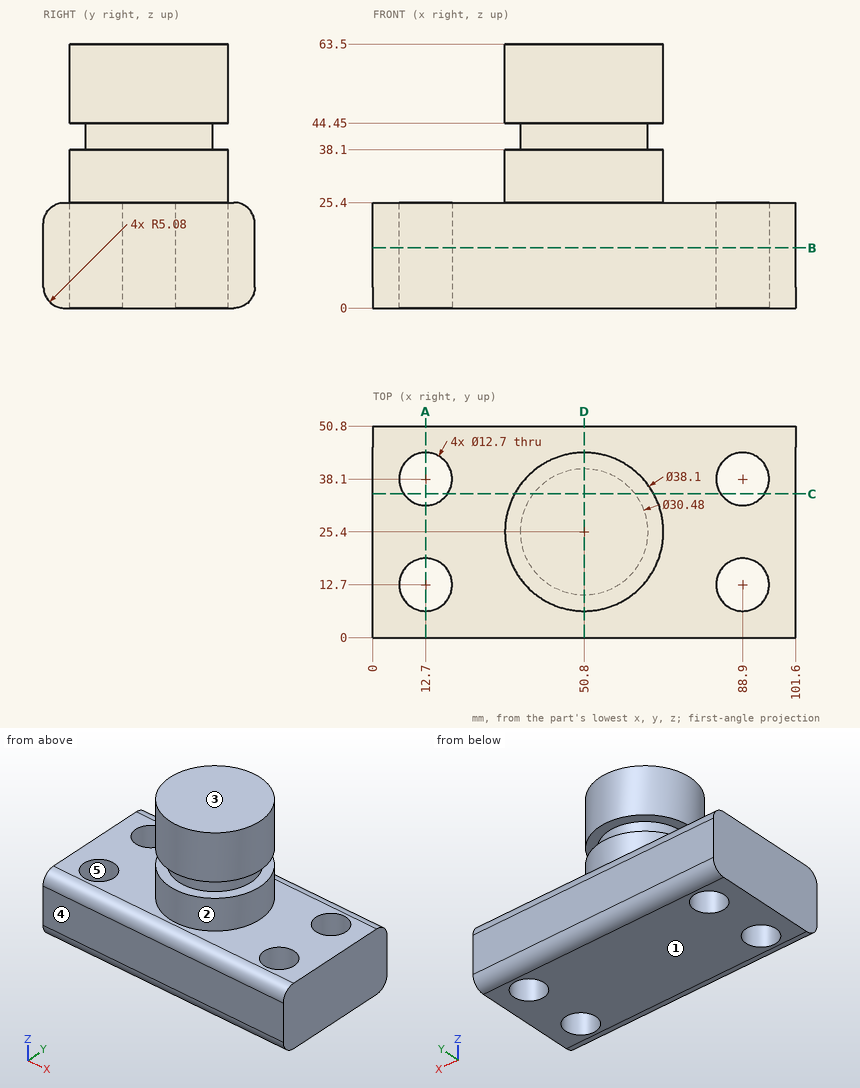
Drawing for the job (mm, zero at the part's lowest x, y, z). A direction names the side the tool comes from. Coordinates: 2 decimals unless noted, no trailing zeros. Order: outer loops, then holes, each group sorted by start corner. A loop starts at its lowest first (then second) coordinate and runs counter-clockwise, first axis right, second up.
Item 1: Band-saw the part on B-B on z = 14.5. List the corners of the cut face in (x, y).
Check sheet entries:
outline: (0, 0) - (101.6, 0) - (101.6, 50.8) - (0, 50.8) - close; hole circle Ø12.7 at (12.7, 12.7); hole circle Ø12.7 at (12.7, 38.1); hole circle Ø12.7 at (88.9, 12.7); hole circle Ø12.7 at (88.9, 38.1)
Item 2: Band-saw the part on A-A on x = 12.7. List the corners of the cut face in (y, z), plus the area to 3 significant figures.
Check sheet entries:
outline: (0, 5.08) arc R5.08 ccw to (5.08, 0) - (6.35, 0) - (6.35, 25.4) - (5.08, 25.4) arc R5.08 ccw to (0, 20.32) - close; (19.05, 0) - (31.75, 0) - (31.75, 25.4) - (19.05, 25.4) - close; (44.45, 0) - (45.72, 0) arc R5.08 ccw to (50.8, 5.08) - (50.8, 20.32) arc R5.08 ccw to (45.72, 25.4) - (44.45, 25.4) - close
area: 623 mm2
Item 3: Band-saw the part on D-D on x = 50.8. List the corners of the cut face in (y, z).
Check sheet entries:
outline: (0, 5.08) arc R5.08 ccw to (5.08, 0) - (45.72, 0) arc R5.08 ccw to (50.8, 5.08) - (50.8, 20.32) arc R5.08 ccw to (45.72, 25.4) - (44.45, 25.4) - (44.45, 38.1) - (40.64, 38.1) - (40.64, 44.45) - (44.45, 44.45) - (44.45, 63.5) - (6.35, 63.5) - (6.35, 44.45) - (10.16, 44.45) - (10.16, 38.1) - (6.35, 38.1) - (6.35, 25.4) - (5.08, 25.4) arc R5.08 ccw to (0, 20.32) - close
Item 4: Two-plate mould, pull along Y, no slides. Class the marked faces 3, 4 and 5: +Y half, -Y half, draft (parallel to the pull), parting line (faces both ways), or undercut.
Check sheet entries:
face 3: draft
face 4: -Y half
face 5: undercut
Item 5: Pin check, flat tips, straight feed: pin 1 Ø1.5 at (x, z) = (36.5, 38) entering from -Y; pin 2 Ø5 at (x, z) = (19.5, 27) entering from -Y; pin 3 Ø8 at (y, z) = (40.5, 35.5) entering from +X. Stop position of each tip, or through.
Check sheet entries:
pin 1: stops at y = 12.01
pin 2: stops at y = 2.19
pin 3: stops at x = 66.28
Item 6: 3-axis set-ups, long thin cutter, end or side, ignore diameter. For the marked faces 1 and 2: which of +Z, -Z, +X, -X, +Y, -Y reach the whole face in a straight line?
Check sheet entries:
face 1: -Z, +X, -X, +Y, -Y
face 2: +Z
Item 7: Band-saw the part on C-C on y = 34.5. List the corners of the cut face in (x, z).
Check sheet entries:
outline: (0, 0) - (7.47, 0) - (7.47, 25.4) - (0, 25.4) - close; (17.93, 0) - (83.67, 0) - (83.67, 25.4) - (67.54, 25.4) - (67.54, 38.1) - (63.02, 38.1) - (63.02, 44.45) - (67.54, 44.45) - (67.54, 63.5) - (34.06, 63.5) - (34.06, 44.45) - (38.58, 44.45) - (38.58, 38.1) - (34.06, 38.1) - (34.06, 25.4) - (17.93, 25.4) - close; (94.13, 0) - (101.6, 0) - (101.6, 25.4) - (94.13, 25.4) - close
Item 8: Drill centre lines: L1, parallel to Y at x = 88, z = 9; L2, parallel to Z at x = 31.5, y = 35; L3, parallel to X at y = 12, z = 9. Where is each one in solid material? Low to high.
Check sheet entries:
L1: y = 0 to 6.41, 18.99 to 31.81, 44.39 to 50.8
L2: z = 0 to 25.4
L3: x = 0 to 6.39, 19.01 to 82.59, 95.21 to 101.6
